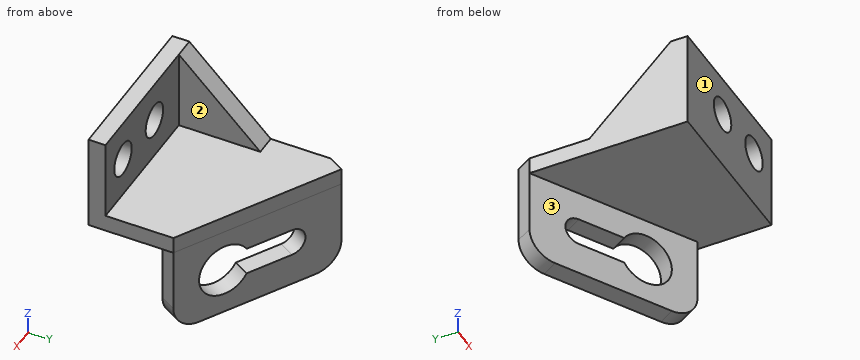
from build123d import *

# Parameters (mm, degrees)
EXTRUDE_1_DEPTH          = 72
EXTRUDE_START            = -7.5
EXTRUDE_1_2_DEPTH        = 7.5
SKETCH_3_W               = 83.138438763
SKETCH_3_H               = 48
EXTRUDE_2_DEPTH          = 7.9375
CUT_EXTRUDE_3_DEPTH      = 113.294938278
CUT_EXTRUDE_3_DEPTH_BACK = 113.294938278
FILLET_1_R               = 12
RIB_1_REACH              = 112.849
SKETCH_5_WALL_W          = 274.608976958
SKETCH_5_WALL_H          = 9
SKETCH_6_R               = 7.5
CUT_EXTRUDE_4_DEPTH      = 111.848644356


# Read off the part's stored shape, not the designer's step: 伸長1
with BuildPart() as part:
    # 草圖1 → Extrude 1 (new body)
    with BuildSketch(Plane(origin=(0, 0, 0), x_dir=(0, 0, -1), z_dir=(1, 0, 0))):
        Polygon((-36, 0), (0, 0), (0, 30), (7.5, 30), (7.5, -7.5), (-36, -7.5), align=None)
    extrude(amount=EXTRUDE_1_DEPTH)

    # Extrude 1 2 outline → Extrude 1 2 (add)
    with BuildSketch(Plane.XY.offset(EXTRUDE_START)):
        Polygon((72, 30), (0, 71.569219382), (0, 30), align=None)
    extrude(amount=EXTRUDE_1_2_DEPTH)

    # 草圖3 → 伸長2 (add)
    with BuildSketch(Plane(origin=(30.990381057, 53.676914536, 0), x_dir=(0.866025403784438, -0.5000000000000011, 0), z_dir=(0.5000000000000011, 0.8660254037844382, 0))):
        with Locations((5.784609691, 24)):
            Rectangle(SKETCH_3_W, SKETCH_3_H)
        with BuildLine():
            Line((-8.146170928, 33.25), (13.109928448, 33.25))
            ThreePointArc((13.109928448, 33.25), (35.353829072, 27), (13.109928448, 20.75))
            Line((13.109928448, 20.75), (-8.146170928, 20.75))
            ThreePointArc((-8.146170928, 20.75), (-14.396170928, 27), (-8.146170928, 33.25))
        make_face(mode=Mode.SUBTRACT)
    extrude(amount=-EXTRUDE_2_DEPTH)

    # 草圖4 → 伸長3 (cut, two sides: drawn at the far end of the back side and taken through both)
    with BuildSketch(Plane.XY.offset(-CUT_EXTRUDE_3_DEPTH_BACK)):
        Polygon((-110.576347035, -129.120067321), (0, 62.403783858), (8.212239163, 76.627799333), (118.788586198, 268.151650512), (-264.259116161, 489.304344581), (-493.624049393, 92.032626748), align=None)
    extrude(amount=CUT_EXTRUDE_3_DEPTH + CUT_EXTRUDE_3_DEPTH_BACK, mode=Mode.SUBTRACT)

    # 圓角1
    fillet_1_edges = [part.edges().sort_by_distance(p)[0] for p in [
        (70.015625, 26.562961679, -48),
        (1.984375, 65.84082218, -48),
    ]]
    fillet(fillet_1_edges, radius=FILLET_1_R)

    # 草圖5 wall → 肋材1 (add, up to next)
    with BuildSketch(Plane(origin=(0, 18, 18), x_dir=(0, -0.707106781187, 0.707106781187), z_dir=(0, 0.707106781187, 0.707106781187)), mode=Mode.PRIVATE) as rib_1_sk1:
        with Locations((0, 4.5)):
            Rectangle(SKETCH_5_WALL_W, SKETCH_5_WALL_H)
    rib_1_tool1 = extrude(rib_1_sk1.sketch, amount=-RIB_1_REACH, mode=Mode.PRIVATE) - part.part
    add(rib_1_tool1.solids().sort_by_distance((0, 18, 18))[0])

    # 草圖6 → 伸長4 (cut, through all)
    with BuildSketch(Plane(origin=(0, 0, 0), x_dir=(1, 0, 0), z_dir=(0, 1, 0))):
        with Locations(Location((57, -18, 0), (0, 0, 270))):
            Circle(SKETCH_6_R)
        with Locations(Location((30, -18, 0), (0, 0, 270))):
            Circle(SKETCH_6_R)
    extrude(amount=-CUT_EXTRUDE_4_DEPTH, mode=Mode.SUBTRACT)


solid = part.part
Design review of the part built by this model. Coordinates are the model's own, in mm. Face numbers are marked on the shaded views. A direction names the side the tool comes from. Round coordinates to 2 decimals unless told otherwise and drop trailing zeros. Write each loop counter-clockwise with the first axis right and the second up, starting at its lowest first coordinate (ties: lowest second). Pieces come first, ordered by that corner, then holes. Notation, with made-up numbers: M -5.75,30.5 L 33.25,30.5 A27 cw 33.25,50.5 Z; hole C -35,21 d11. An arc over 180 degrees is marked long. One line per item, written item: value. Start each with the question number.
1. Clearance check with flat-ended pins moving along their axes: P1, Ø1.5, axis at x = 15, y = 41.5, coming from the +Z side; P2, Ø12, axis at x = 14, z = -39, coming from the +Y side; P3, Ø1.5, axis at y = 37, z = -17.5, coming from the +X side. State where each tip first meets the part, or that it passes through.
2. To check wall thickness, follow probe 1 along X at (y, z) = (-5, 18); probe 2 along Z at (x, y) = (37.5, 26.5). State the ranges of each line that lie inside material, in increasing order. Write a range as from..to.
3. Take a section at C-C on x = 30. State the section outline as (y, z) points.
4. Take a section at A-A on z = 13. State the section outline as (x, y) points.
5. Take a section at D-D on z = -30.5. State the section outline as (x, y) points, then the cut area to 3 significant figures.
6. For the marked faces 1, 2 and 3, list the 3-axis set-ups (+Z, -Z, +X, -X, +Y, -Y) from which the entire face can be reached by the end or side of a thin tool; tool diameter is ignored.
7. Take a section at B-B on z = -17. State the section outline as (x, y) points, then the cut area to 3 significant figures.
Computed:
1. P1: stops at z = 0
1. P2: stops at y = 66.95
1. P3: stops at x = 61.17
2. probe 1: x = 0..22.5, 37.5..49.5, 64.5..72
2. probe 2: z = -7.5..0
3. outline: M -7.5,-7.5 L 45.08,-7.5 L 45.08,-20.75 L 54.25,-20.75 L 54.25,0 L 0,0 L 0,10.5 L -7.5,10.5 Z; M -7.5,25.5 L 0,25.5 L 0,36 L -7.5,36 Z; M 45.08,-48 L 54.25,-48 L 54.25,-33.25 L 45.08,-33.25 Z
4. outline: M 0,-7.5 L 24.41,-7.5 L 24.41,0 L 9,0 L 9,23 L 0,23 Z; M 35.59,-7.5 L 51.41,-7.5 L 51.41,0 L 35.59,0 Z; M 62.59,-7.5 L 72,-7.5 L 72,0 L 62.59,0 Z
5. outline: M 0,62.4 L 15.48,53.46 L 19.45,60.34 L 3.97,69.28 Z; M 57.19,29.39 L 68.03,23.13 L 72,30 L 61.16,36.26 Z
5. area: 241 mm²
6. face 1: +Z, -Z, +X, -X, -Y
6. face 2: +Z, +X, +Y
6. face 3: -Z, -X, -Y
7. outline: M 0,62.4 L 41.5,38.44 L 45.47,45.32 L 3.97,69.28 Z; M 52.99,31.81 L 68.03,23.13 L 72,30 L 56.96,38.68 Z
7. area: 518 mm²
